```python
from build123d import *

# Parameters (mm, degrees)
SKETCH1_W           = 17.3
SKETCH1_H           = 5.8
BOSS_EXTRUDE1_DEPTH = 7
SKETCH3_W           = 15
SKETCH3_H           = 4.9
CUT_EXTRUDE1_DEPTH  = 5
SKETCH4_W           = 1.2
SKETCH4_H           = 3.5
CUT_EXTRUDE2_DEPTH  = 4
SKETCH5_W           = 17.3
SKETCH5_H           = 0.8
CUT_EXTRUDE3_DEPTH  = 0.8
SKETCH6_W           = 0.8
SKETCH6_H           = 0.8
CUT_EXTRUDE4_DEPTH  = 10
SKETCH7_W           = 15
SKETCH7_H           = 1
CUT_EXTRUDE5_DEPTH  = 0.3


with BuildPart() as part:
    # Sketch1 → Boss-Extrude1 (new body)
    with BuildSketch(Plane(origin=(0, 0, 0), x_dir=(1, 0, 0), z_dir=(0, 1, 0))):
        Rectangle(SKETCH1_W, SKETCH1_H)
    extrude(amount=BOSS_EXTRUDE1_DEPTH)

    # Sketch3 → Cut-Extrude1 (cut)
    with BuildSketch(Plane.XZ):
        Rectangle(SKETCH3_W, SKETCH3_H)
    extrude(amount=-CUT_EXTRUDE1_DEPTH, mode=Mode.SUBTRACT)

    # Sketch4 → Cut-Extrude2 (cut)
    with BuildSketch(Plane.XY.offset(2.9)):
        with Locations((-5.4, 1.75)):
            Rectangle(SKETCH4_W, SKETCH4_H)
        with Locations((5.4, 1.75)):
            Rectangle(SKETCH4_W, SKETCH4_H)
    extrude(amount=-CUT_EXTRUDE2_DEPTH, mode=Mode.SUBTRACT)

    # Sketch5 → Cut-Extrude3 (cut)
    with BuildSketch(Plane(origin=(0, 7, 0), x_dir=(1, 0, 0), z_dir=(0, 1, 0))):
        with Locations((0, 2.5)):
            Rectangle(SKETCH5_W, SKETCH5_H)
    extrude(amount=-CUT_EXTRUDE3_DEPTH, mode=Mode.SUBTRACT)

    # Sketch6 → Cut-Extrude4 (cut)
    with BuildSketch(Plane(origin=(0, 7, 0), x_dir=(1, 0, 0), z_dir=(0, 1, 0))):
        with Locations((5.8, -0.55)):
            Rectangle(SKETCH6_W, SKETCH6_H)
        with Locations((3.866666667, -0.55)):
            Rectangle(SKETCH6_W, SKETCH6_H)
        with Locations((1.933333333, -0.55)):
            Rectangle(SKETCH6_W, SKETCH6_H)
        with Locations((0, -0.55)):
            Rectangle(SKETCH6_W, SKETCH6_H)
        with Locations((-1.933333333, -0.55)):
            Rectangle(SKETCH6_W, SKETCH6_H)
        with Locations((-3.866666667, -0.55)):
            Rectangle(SKETCH6_W, SKETCH6_H)
        with Locations((-5.8, -0.55)):
            Rectangle(SKETCH6_W, SKETCH6_H)
    extrude(amount=-CUT_EXTRUDE4_DEPTH, mode=Mode.SUBTRACT)

    # Sketch7 → Cut-Extrude5 (cut)
    with BuildSketch(Plane.XZ.offset(-5)):
        with Locations((0, -1.95)):
            Rectangle(SKETCH7_W, SKETCH7_H)
    extrude(amount=-CUT_EXTRUDE5_DEPTH, mode=Mode.SUBTRACT)


solid = part.part
```
Here's how the part is built. I have some questions about the finished solid (model axes, mm). A direction names the side the tool comes from. Round coordinates to 2 decimals unless told otherwise and drop trailing zeros. Loops run counter-clockwise (first coordinate to the right, second up) from the corner with the lowest first, then second, coordinate; pieces in that order, holes last. Notation, with made-up numbers: (-34, 45) -> (-21, 45) arc R27 ccw to (-21, 79) -> close; hole circle Ø4 at (51, 16). An arc over 180 degrees is marked (long way). Answer as CSV lines item,"result".
1. If I drill on L1, parallel to X at y = 1, z = -0.8; L2, parallel to Z at x = -2.25, y = 6.5; L3, parallel to Z at x = 0.75, y = 3.25, over which ranges is the centre line in solid material (lowest first)?
Final values:
L1,"x = -8.65 to -7.5, 7.5 to 8.65"
L2,"z = -2.1 to 0.15, 0.95 to 2.9"
L3,"z = -2.9 to -2.45, 2.45 to 2.9"
2. If we section it at C-C on y = 6: Count the separate pieces of the cut face and the enclosed holes in it, plus the area to 3 significant figures.
Final values:
separate pieces,"1"
enclosed holes,"7"
area,"95.9 mm^2"
3. Which directions (+Z, -Z, +X, -X, +Y, -Y) give clear straight access to the entire face, cutting with the end or side of a thin tool? Please do faces 5 (the face through (6, 6, 0.15)), 6 (the face through (-7.5, 3, 0)), 7 (the face through (0, 3, -2.9)).
Final values:
face 5,"+Y, -Y"
face 6,"-Y"
face 7,"-Z, +X, -X, +Y, -Y"
4. If we section it at D-D on z = -1.7: Please give me the cut outline in (x, y), plus the area to 3 significant figures.
Final values:
outline,"(-8.65, 0) -> (-7.5, 0) -> (-7.5, 5.3) -> (7.5, 5.3) -> (7.5, 0) -> (8.65, 0) -> (8.65, 7) -> (-8.65, 7) -> close"
area,"41.6 mm^2"
5. If we section it at A-A on x = -1.75: Please give me the cut outline in (y, z), plus the area to 3 significant figures.
Final values:
outline,"(0, -2.9) -> (6.2, -2.9) -> (6.2, -2.1) -> (7, -2.1) -> (7, 0.15) -> (5, 0.15) -> (5, -1.45) -> (5.3, -1.45) -> (5.3, -2.45) -> (0, -2.45) -> close; (0, 2.45) -> (5, 2.45) -> (5, 0.95) -> (7, 0.95) -> (7, 2.9) -> (0, 2.9) -> close"
area,"13.6 mm^2"
6. For pin 1 (0.5 mm diameter, centred on x = 5.5, z = 2.5, fed in from -Y), with a flat end and sliding along its axis, tell me the tip position at first contact or that it passes through.
Final values:
pin 1,"stops at y = 3.5"
7. If we section it at B-B on y = 1.5: Please give me the cut outline in (x, z).
Final values:
outline,"(-8.65, -2.9) -> (8.65, -2.9) -> (8.65, 2.9) -> (6, 2.9) -> (6, 2.45) -> (7.5, 2.45) -> (7.5, -2.45) -> (-7.5, -2.45) -> (-7.5, 2.45) -> (-6, 2.45) -> (-6, 2.9) -> (-8.65, 2.9) -> close; (-4.8, 2.45) -> (4.8, 2.45) -> (4.8, 2.9) -> (-4.8, 2.9) -> close"
8. Thinking about a two-plate mould opening in X: for faces 1 (the face through (-8.65, 3, 0)), 2 (the face through (-6, 6, 0.15)), 3 (the face through (8.65, 3, 0)), 4 (the face through (0, 2, 2.45)), which applies, released by +X, released by -X, zero draft, split by the parting line, or undercut?
Final values:
face 1,"released by -X"
face 2,"undercut"
face 3,"released by +X"
face 4,"undercut"
